Input: part model. Units: mm. Frame: model coordinates. Face numbers are marked on the shaded views. A direction names the side the tool comes from. Round coordinates to 2 decimals unless told otherwise and drop trailing zeros. Loops run counter-clockwise (first coordinate to the right, second up) from the corner with the lowest first, then second, coordinate; pieces in that order, holes last. Notation, with made-up numbers: (89, 75) -> (146, 75) arc R14 cw to (146, 84) -> close; hole circle Ø3 at (39.25, -31). An arc over 180 degrees is marked (long way). Answer as a JSON object with one key per item and string values. Group by question number.
Item 1: Material intervals for line 1 (Z direction, x = -1.25, y = 1); line 2 (Z direction, x = 1.75, y = -0.5); line 3 (Y direction, x = 0.75, z = 31), sorted ascending. Write a range as [from, to].
Item 2: Set-up query: the marked faces 1 and 2. Return all of +Z, -Z, +X, -X, +Y, -Y with unobstructed straight access to the full face (end or side cutting, diameter ignored); none if empty.
Item 3: Section query A-A on z = 47. Return loops of the section in (x, y), and give its area (3 significant figures).
Item 4: Pin query (flat end, axial travel): pin 1 (2 mm diameter, centred on y = 2, z = 19, fed in from -X); pin 2 (1 mm diameter, centred on y = 1, z = 41.5, fed in from -X). Return the tip coordinate at first contact, or that it passes through.
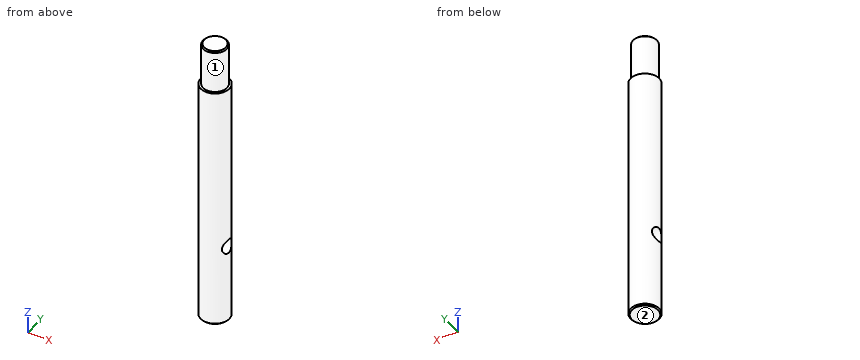
from build123d import *

# Parameters (mm, degrees)
SKETCH1_R             = 3
BOSS_EXTRUDE1_DEPTH   = 52
SKETCH2_R             = 2.5
BOSS_EXTRUDE2_DEPTH   = 9
CHAMFER1_SIZE         = 0.25
CHAMFER2_SIZE         = 0.25
F_3_0MM_DOWEL_HOLE1_D = 3


with BuildPart() as part:
    # Sketch1 → Boss-Extrude1 (new body)
    with BuildSketch(Plane.XY):
        with Locations(Location((0, 0, 0), (0, 0, 180))):
            Circle(SKETCH1_R)
    extrude(amount=BOSS_EXTRUDE1_DEPTH)

    # Sketch2 → Boss-Extrude2 (add)
    with BuildSketch(Plane.XY.offset(52)):
        Circle(SKETCH2_R)
    extrude(amount=BOSS_EXTRUDE2_DEPTH)

    # Chamfer1
    chamfer1_edges = [part.edges().sort_by_distance(p)[0] for p in [
        (-2.5, 0, 61),
    ]]
    chamfer(chamfer1_edges, length=CHAMFER1_SIZE)

    # Chamfer2
    chamfer2_edges = [part.edges().sort_by_distance(p)[0] for p in [
        (3, 0, 0),
    ]]
    chamfer(chamfer2_edges, length=CHAMFER2_SIZE)

    # Ø3.0mm Dowel Hole1 (through all)
    with Locations(Plane(origin=(2.990601236, -0.237285162, 16.733200531), x_dir=(0.079095054135, 0.996867078607, 0), z_dir=(0.996867078607, -0.079095054135, 0))):
        with Locations((0, 0)):
            Hole(F_3_0MM_DOWEL_HOLE1_D / 2)


solid = part.part
Solved:
{
 "1": {"line 1": "[0, 15.53], [17.93, 61]", "line 2": "[0, 15.28], [18.19, 61]", "line 3": "[-2.9, 2.9]"},
 "2": {"face 1": "+Z", "face 2": "-Z, +X, -X, +Y, -Y"},
 "3": {"outline": "circle Ø6 at (0, 0)", "area": "28.3 mm²"},
 "4": {"pin 1": "x = -2.83", "pin 2": "x = -2.96"}
}
